from build123d import *

# Parameters (mm, degrees)
F1_DEPTH = 203.2
F2_R     = 6.35
F3_DEPTH = 50.8
F4_R     = 6.35
F5_DEPTH = 25.4


with BuildPart() as f1:
    # F0 (on Front) → F1 (new body)
    with BuildSketch(Plane.XZ):
        with BuildLine():
            Line((-19.05, -25.4), (19.05, -25.4))
            ThreePointArc((19.05, -25.4), (23.540128, -23.540128), (25.4, -19.05))
            Line((25.4, -19.05), (25.4, 19.05))
            ThreePointArc((25.4, 19.05), (23.540128, 23.540128), (19.05, 25.4))
            Line((19.05, 25.4), (-19.05, 25.4))
            ThreePointArc((-19.05, 25.4), (-23.540128, 23.540128), (-25.4, 19.05))
            Line((-25.4, 19.05), (-25.4, -19.05))
            ThreePointArc((-25.4, -19.05), (-23.540128, -23.540128), (-19.05, -25.4))
        make_face()
        with BuildLine():
            ThreePointArc((19.05, -12.7), (17.190128, -17.190128), (12.7, -19.05))
            Line((12.7, -19.05), (-12.7, -19.05))
            ThreePointArc((-12.7, -19.05), (-17.190128, -17.190128), (-19.05, -12.7))
            Line((-19.05, -12.7), (-19.05, 12.7))
            ThreePointArc((-19.05, 12.7), (-17.190128, 17.190128), (-12.7, 19.05))
            Line((-12.7, 19.05), (12.7, 19.05))
            ThreePointArc((12.7, 19.05), (17.190128, 17.190128), (19.05, 12.7))
            Line((19.05, 12.7), (19.05, -12.7))
        make_face(mode=Mode.SUBTRACT)
    extrude(amount=F1_DEPTH)

    # F2 (on face) → F3 (cut)
    with BuildSketch(Plane.YZ.offset(25.4)):
        with Locations((-101.6, 0)):
            Circle(F2_R)
    extrude(amount=-F3_DEPTH, mode=Mode.SUBTRACT)

    # F4 (on face) → F5 (cut)
    with BuildSketch(Plane.XY.offset(25.4)):
        with Locations((0, -177.8)):
            Circle(F4_R)
    extrude(amount=-F5_DEPTH, mode=Mode.SUBTRACT)


solid = f1.part
Geometry check sheet. Reference: the model listing, model coordinates, mm. A direction names the side the tool comes from. Round coordinates to 2 decimals unless told otherwise and drop trailing zeros. Order: outer loops, then holes, each group sorted by start corner. A loop starts at its lowest first (then second) coordinate and runs counter-clockwise, first axis right, second up. Notation, with made-up numbers: (68.5, 23) -> (117.5, 23) arc R11 ccw to (117.5, 32) -> close; hole circle Ø10 at (9.5, 63). An arc over 180 degrees is marked (long way). Use one line per item in the form item = value.
1. Cross-section at A-A, the plane x = 0. Enter the section's corners in (y, z).
Working result:
outline = (-203.2, -25.4) -> (0, -25.4) -> (0, -19.05) -> (-203.2, -19.05) -> close; (-203.2, 19.05) -> (-184.15, 19.05) -> (-184.15, 25.4) -> (-203.2, 25.4) -> close; (-171.45, 19.05) -> (0, 19.05) -> (0, 25.4) -> (-171.45, 25.4) -> close
2. Cross-section at C-C, the plane z = 0. Enter the section's corners in (x, y).
Working result:
outline = (-25.4, -203.2) -> (-19.05, -203.2) -> (-19.05, -107.95) -> (-25.4, -107.95) -> close; (-25.4, -95.25) -> (-19.05, -95.25) -> (-19.05, 0) -> (-25.4, 0) -> close; (19.05, -203.2) -> (25.4, -203.2) -> (25.4, -107.95) -> (19.05, -107.95) -> close; (19.05, -95.25) -> (25.4, -95.25) -> (25.4, 0) -> (19.05, 0) -> close
3. Cross-section at B-B, the plane x = -10.5. Enter the section's corners in (y, z), plus the area to 3 significant figures.
Working result:
outline = (-203.2, -25.4) -> (0, -25.4) -> (0, -19.05) -> (-203.2, -19.05) -> close; (-203.2, 19.05) -> (0, 19.05) -> (0, 25.4) -> (-203.2, 25.4) -> close
area = 2,580 mm^2
4. Go/stop test with flat-tipped pins: pin 1 (10 mm diameter, centred on y = -101.6, z = 0, fed in from +X); pin 2 (6 mm diameter, centred on x = 19.5, z = -4, fed in from +Y). Record where each tip stops, or that it passes through.
Working result:
pin_1 = through
pin_2 = 0
5. Cross-section at D-D, the plane y = -101.6. Enter the section's corners in (x, z).
Working result:
outline = (-25.4, -19.05) arc R6.35 ccw to (-19.05, -25.4) -> (19.05, -25.4) arc R6.35 ccw to (25.4, -19.05) -> (25.4, -6.35) -> (19.05, -6.35) -> (19.05, -12.7) arc R6.35 cw to (12.7, -19.05) -> (-12.7, -19.05) arc R6.35 cw to (-19.05, -12.7) -> (-19.05, -6.35) -> (-25.4, -6.35) -> close; (-25.4, 6.35) -> (-19.05, 6.35) -> (-19.05, 12.7) arc R6.35 cw to (-12.7, 19.05) -> (12.7, 19.05) arc R6.35 cw to (19.05, 12.7) -> (19.05, 6.35) -> (25.4, 6.35) -> (25.4, 19.05) arc R6.35 ccw to (19.05, 25.4) -> (-19.05, 25.4) arc R6.35 ccw to (-25.4, 19.05) -> close
6. Mould release check, pull along Y, two halves, no side actions. Record for faces 1 (the face through (0, 0, 23)), 2 (the face through (0, -203.2, 23)), 3 (the face through (22.269, -107.944, 0.279)), 4 (the face through (-23.49, -100.18, 23.59)): pulls with the +Y half, pulls with the -Y half, needs draft (parallel to the pull), parting line crosses it, or undercut.
Working result:
face_1 = pulls with the +Y half
face_2 = pulls with the -Y half
face_3 = undercut
face_4 = needs draft
7. Set-up check for faces 5 (the face through (0, -100, 25.4)), 6 (the face through (-17.14, -100.18, -17.24)): record each of +Z, -Z, +X, -X, +Y, -Y from which the full face is reachable in a straight line by a thin tool's end or side.
Working result:
face_5 = +Z, +X, -X, +Y, -Y
face_6 = +Y, -Y
8. Scan lines: line 1 along Z through (x, y) = (-3.5, -73.5); line 2 along Y through (x, z) = (0, 21). Record each from-to range of solid material in increasing order. Write a range as from..to.
Working result:
line_1 = -25.4..-19.05, 19.05..25.4
line_2 = -203.2..-184.15, -171.45..0
